Work out the finished part from the listing and answer in its coordinate system (mm). Face numbers are marked on the shaded views. A direction names the side the tool comes from. Round coordinates to 2 decimals unless told otherwise and drop trailing zeros. Order: outer loops, then holes, each group sorted by start corner. A loop starts at its lowest first (then second) coordinate and runs counter-clockwise, first axis right, second up. Notation, with made-up numbers: (42, -13) -> (93, -13) arc R27 cw to (93, 4) -> close; hole circle Ø11 at (-2.75, 65.5). An arc over 180 degrees is marked (long way). Use one line per item in the form item = value.
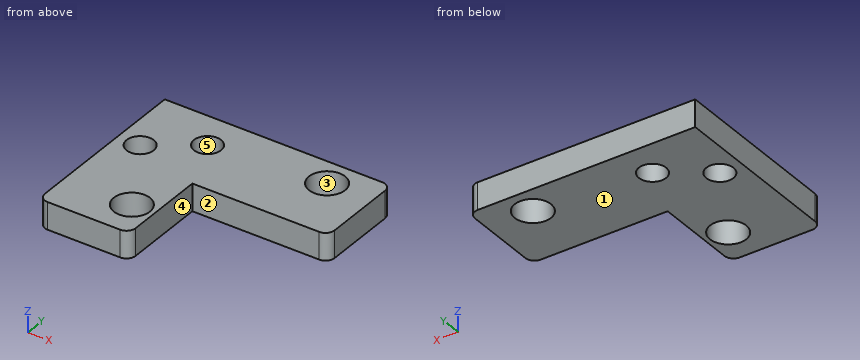
```python
from build123d import *

# Parameters (mm, degrees)
SKETCH_1_W          = 25
SKETCH_1_H          = 10
EXTRUDE_1_DEPTH     = 3
SKETCH_2_R          = 1.5
CUT_EXTRUDE_1_DEPTH = 3
SKETCH_3_R          = 2
CUT_EXTRUDE_2_DEPTH = 10
SKETCH_4_W          = 10
SKETCH_4_H          = 10
EXTRUDE_2_DEPTH     = 3
SKETCH_5_R          = 2
CUT_EXTRUDE_3_DEPTH = 3
FILLET_1_R          = 1


with BuildPart() as part:
    # 草图1 → 凸台-拉伸1 (new body)
    with BuildSketch(Plane.XY):
        with Locations((12.5, 5)):
            Rectangle(SKETCH_1_W, SKETCH_1_H)
    extrude(amount=EXTRUDE_1_DEPTH)

    # 草图2 → 切除-拉伸1 (cut)
    with BuildSketch(Plane.XY.offset(3)):
        with Locations((2.5, 2.5)):
            Circle(SKETCH_2_R)
        with Locations((7.5, 6)):
            Circle(SKETCH_2_R)
    extrude(amount=-CUT_EXTRUDE_1_DEPTH, mode=Mode.SUBTRACT)

    # 草图3 → 切除-拉伸2 (cut)
    with BuildSketch(Plane.XY.offset(3)):
        with Locations((20, 7)):
            Circle(SKETCH_3_R)
    extrude(amount=-CUT_EXTRUDE_2_DEPTH, mode=Mode.SUBTRACT)

    # 草图4 → 凸台-拉伸2 (add)
    with BuildSketch(Plane.XY.offset(3)):
        with Locations((5, -5)):
            Rectangle(SKETCH_4_W, SKETCH_4_H)
    extrude(amount=-EXTRUDE_2_DEPTH)

    # 草图5 → 切除-拉伸3 (cut)
    with BuildSketch(Plane.XY.offset(3)):
        with Locations((7.5, -6)):
            Circle(SKETCH_5_R)
    extrude(amount=-CUT_EXTRUDE_3_DEPTH, mode=Mode.SUBTRACT)

    # 圆角1
    fillet_1_edges = [part.edges().sort_by_distance(p)[0] for p in [
        (0, -10, 1.5),
        (10, -10, 1.5),
        (25, 10, 1.5),
        (25, 0, 1.5),
    ]]
    fillet(fillet_1_edges, radius=FILLET_1_R)


solid = part.part
```
Item 1: Flat-ended cylindrical pins translate along their axes: P1, Ø0.9, axis at x = 16, z = 1, coming from the -Y side; P2, Ø3, axis at x = 7.5, y = -6, coming from the +Z side. Find the tip coordinate at first contact, or state that the pin passes through.
Findings:
P1 = 0
P2 = through
Item 2: The part is cut by section B-B, the plane x = 7.5. Give the vertices of the cut face in (y, z).
Findings:
outline = (-10, 0) -> (-8, 0) -> (-8, 3) -> (-10, 3) -> close; (-4, 0) -> (4.5, 0) -> (4.5, 3) -> (-4, 3) -> close; (7.5, 0) -> (10, 0) -> (10, 3) -> (7.5, 3) -> close
Item 3: The part is cut by section C-C, the plane z = 2.4. Give the vertices of the cut face in (x, y).
Findings:
outline = (0, -9) arc R1 ccw to (1, -10) -> (9, -10) arc R1 ccw to (10, -9) -> (10, 0) -> (24, 0) arc R1 ccw to (25, 1) -> (25, 9) arc R1 ccw to (24, 10) -> (0, 10) -> close; hole circle Ø3 at (2.5, 2.5); hole circle Ø4 at (7.5, -6); hole circle Ø3 at (7.5, 6); hole circle Ø4 at (20, 7)
Item 4: For the marked faces 4 and 5, determine the directions among +Z, -Z, +X, -X, +Y, -Y from which every point of the face is accessible in a straight line to the end or side of a thin tool.
Findings:
face_4 = +Z, -Z, +X, -Y
face_5 = +Z, -Z
Item 5: Determine the mould class of the marked faces 1, 2 and 3 for opening direction Y: released by +Y, released by -Y, zero draft, split by the parting line, or undercut.
Findings:
face_1 = zero draft
face_2 = released by -Y
face_3 = undercut
Item 6: The part is cut by section A-A, the plane y = -6. Give the vertices of the cut face in (x, z).
Findings:
outline = (0, 0) -> (5.5, 0) -> (5.5, 3) -> (0, 3) -> close; (9.5, 0) -> (10, 0) -> (10, 3) -> (9.5, 3) -> close
Item 7: The part is cut by section D-D, the plane x = 2.5. Give the vertices of the cut face in (y, z), and give its area (3 significant figures).
Findings:
outline = (-10, 0) -> (1, 0) -> (1, 3) -> (-10, 3) -> close; (4, 0) -> (10, 0) -> (10, 3) -> (4, 3) -> close
area = 51.0 mm^2
Item 8: Consider line 1 along Y through (x, z) = (7.5, 0.7); line 2 along Y through (x, z) = (2.5, 2); line 3 along Y through (x, z) = (8, 2.3). Determine where each line is inside the solid, lowest interval first.
Findings:
line_1 = -10 to -8, -4 to 4.5, 7.5 to 10
line_2 = -10 to 1, 4 to 10
line_3 = -10 to -7.94, -4.06 to 4.59, 7.41 to 10
